```python
from build123d import *

# Parameters (mm, degrees)
F1_DEPTH = 8
F2_W     = 45
F2_H     = 8
F3_DEPTH = 5
F4_T     = -5
F5_D     = 2.8
F5_DEPTH = 11
F5_TIP   = 0.8412048666
F7_DEPTH = 8
F9_D     = 4.1
F9_DEPTH = 7
F9_TIP   = 1.231764269
F10_R    = 5


with BuildPart() as f1:
    # F0 (on Top) → F1 (new body)
    with BuildSketch(Plane.XY):
        Polygon((81.39341741, -55.7623273981), (16.39341741, 9.2376726019), (16.39341741, -55.7623273981), align=None)
    extrude(amount=F1_DEPTH)

    # F2 (on face) → F3 (cut)
    with BuildSketch(Plane(origin=(12.8155450059, 12.8155450059, 0), x_dir=(-0.7071067812, 0.7071067812, 0), z_dir=(0.7071067812, 0.7071067812, 0))):
        with Locations((-51.0598756783, 4)):
            Rectangle(F2_W, F2_H)
    extrude(amount=-F3_DEPTH, mode=Mode.SUBTRACT)

    # F4
    f4_openings = [f1.faces().sort_by_distance(p)[0] for p in [
        (36.976212, -35.173116, 8),
        (36.976212, -35.173116, 0),
    ]]
    offset(amount=F4_T, openings=f4_openings, kind=Kind.INTERSECTION)

    # F5
    with Locations(Plane(origin=(12.8155450059, 12.8155450059, 0), x_dir=(-0.7071067812, 0.7071067812, 0), z_dir=(0.7071067812, 0.7071067812, 0))):
        with Locations((-26.0598756783, 4), (-76.0598756783, 4)):
            Hole(F5_D / 2, depth=F5_DEPTH)
            with Locations((0, 0, -(F5_DEPTH + F5_TIP / 2))):  # 118° drill point
                Cone(0, F5_D / 2, F5_TIP, mode=Mode.SUBTRACT)

    # F6 (on face) → F7 (join)
    with BuildSketch(Plane.XY.offset(8)):
        Polygon((21.39341741, -35.7623273981), (16.39341741, -35.7623273981), (16.39341741, -55.7623273981), (21.39341741, -55.7623273981), (21.39341741, -50.7623273981), align=None)
    extrude(amount=F7_DEPTH)

    # F9
    with Locations(Plane(origin=(16.39341741, 0, 0), x_dir=(0, -1, 0), z_dir=(-1, 0, 0))):
        with Locations((44.8939013033, 11.6526295621)):
            Hole(F9_D / 2, depth=F9_DEPTH)
            with Locations((0, 0, -(F9_DEPTH + F9_TIP / 2))):  # 118° drill point
                Cone(0, F9_D / 2, F9_TIP, mode=Mode.SUBTRACT)

    # F10
    f10_edges = [f1.edges().sort_by_distance(p)[0] for p in [
        (16.393417, 9.237673, 4),
        (81.393417, -55.762327, 4),
    ]]
    fillet(f10_edges, radius=F10_R)


solid = f1.part
```
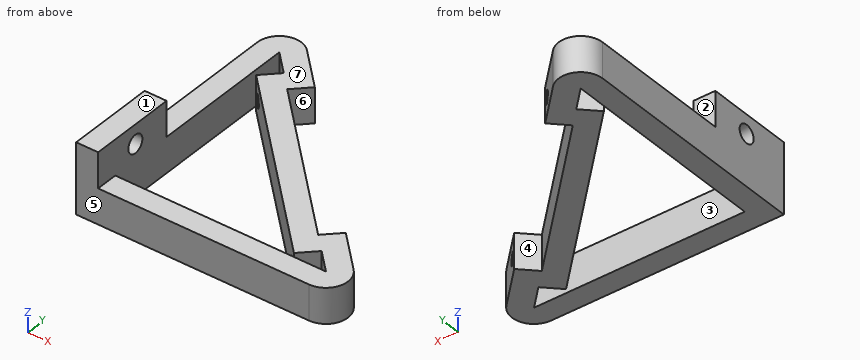
Could you check a few things on this model? Use its own coordinates, in mm. Face numbers are marked on the shaded views. A direction names the side the tool comes from. Round coordinates to 2 decimals unless told otherwise and drop trailing zeros. Order: outer loops, then holes, each group sorted by start corner. A loop starts at its lowest first (then second) coordinate and runs counter-clockwise, first axis right, second up. Notation, with made-up numbers: M -7,34 L 41,34 A16 ccw 41,59 Z; hole C 57,-23.75 d9. An arc over 180 degrees is marked long. One line per question, with ' | ' between items. Start each with the question number.
(1) For the marked faces 4, 5, 6 and 7, which set-ups out of +Z, -Z, +X, -X, +Y, -Y let a thin tool reach every point of the face, with its end or its side?
(2) Suppose I cut it at C-C on y = -28. List the corners of the cut face in (x, z) for me.
(3) Please list where these lines run through material, in increasing order: line 1 along Y through (x, z) = (20, 11.5); line 2 along Z through (x, y) = (50.5, -35); line 3 along Y through (x, z) = (50, 7).
(4) Suppose I cut it at B-B on x = 38.5. List the corners of the cut face in (y, z) for me.
(5) Thinking about a two-plate mould opening in Y: for the marked faces 1, 2 and 3, which applies, +Y half, -Y half, draft (parallel to the pull), parting line (faces both ways), or undercut?
(6) Suppose I cut it at D-D on x = 27. Count the separate pieces of the cut face and the enclosed holes in it, then the cut area to 3 significant figures.
(7) Suppose I cut it at A-A on z = 7. List the corners of the cut face in (x, y) for me.
(8) For P1, Ø6.5, axis at x = 53.5, z = 2.5, coming from the +Y side; P2, Ø6, axis at y = -26.5, z = 2, coming from the +X side; P3, Ø2.5, axis at x = 19, z = 12, coming from the +Y side, each with a flat end and sliding along its axis, tell me the tip position at first contact or that it passes through.
Geometry results:
1) face 4: +Z, -Z, +Y | face 5: +Z, -Z, +X, -X, -Y | face 6: +Z, -Z, +X | face 7: +Z, +X, +Y
2) outline: M 16.39,0 L 21.39,0 L 21.39,8 L 16.39,8 Z; M 39.49,0 L 46.56,0 L 46.56,8 L 39.49,8 Z
3) line 1: -55.76 to -46.94, -42.85 to -35.76 | line 2: 0 to 8 | line 3: -55.76 to -50.76, -38.51 to -31.44
4) outline: M -55.76,0 L -50.76,0 L -50.76,8 L -55.76,8 Z; M -27.01,0 L -19.94,0 L -19.94,8 L -27.01,8 Z
5) face 1: draft | face 2: +Y half | face 3: undercut
6) separate pieces: 2 | enclosed holes: 1 | area: 144 mm²
7) outline: M 16.39,-55.76 L 69.32,-55.76 A5 ccw 72.86,-47.23 L 64.83,-39.2 L 61.29,-42.73 L 29.47,-10.91 L 33.01,-7.38 L 24.93,0.7 A5 ccw 16.39,-2.83 Z; hole M 21.39,-50.76 L 69.32,-50.76 L 64.83,-46.27 L 61.29,-49.81 L 22.4,-10.91 L 25.94,-7.38 L 21.39,-2.83 Z
8) P1: y = -31.69 | P2: x = 48.06 | P3: y = -35.76
